Geometry: final body of the model. Coordinates: model frame, mm. Face numbers are marked on the shaded views. A direction names the side the tool comes from. Round coordinates to 2 decimals unless told otherwise and drop trailing zeros. Loops run counter-clockwise (first coordinate to the right, second up) from the corner with the lowest first, then second, coordinate; pieces in that order, holes last. Notation, with made-up numbers: (16.5, -19.5) - (36.5, -19.5) arc R23 cw to (36.5, 19.5) - close; hole circle Ø10 at (-13, 59). An arc over 180 degrees is marked (long way). Answer in a Markdown table with one row per item. Add a question column.
from build123d import *

# Parameters (mm, degrees)
CROQUIS2_W              = 82
CROQUIS2_H              = 82
CORTAR_EXTRUIR1_DEPTH   = 11.5
SALIENTE_EXTRUIR1_DEPTH = 10.5
CROQUIS4_W              = 14
CROQUIS4_H              = 8.5
CORTAR_EXTRUIR2_DEPTH   = 10.5
CROQUIS5_R              = 1.5
CORTAR_EXTRUIR3_DEPTH   = 10


with BuildPart() as part:
    # Croquis1 → Revolución1 (revolve)
    with BuildSketch(Plane.XY):
        Polygon((-67.901642817, 46.97611702), (-67.901642817, 61.97611702), (-67.901642817, 71.97611702), (-86.901642817, 71.97611702), (-86.901642817, 61.97611702), (-96.901642817, 61.97611702), (-96.901642817, 59.97611702), (-86.901642817, 59.97611702), (-69.901642817, 46.97611702), (-101.901642817, -33.02388298), (-99.901642817, -33.02388298), align=None)
    revolve(axis=Axis((-26.901642817, 46.97611702, 0), (0, -1, 0)))

    # Croquis2 → Cortar-Extruir1 (cut)
    with BuildSketch(Plane(origin=(0, 71.97611702, 0), x_dir=(1, 0, 0), z_dir=(0, 1, 0))):
        with Locations((-26.901642817, 0)):
            Rectangle(CROQUIS2_W, CROQUIS2_H)
    extrude(amount=-CORTAR_EXTRUIR1_DEPTH, mode=Mode.SUBTRACT)

    # Croquis3 → Saliente-Extruir1 (add)
    with BuildSketch(Plane(origin=(0, 71.97611702, 0), x_dir=(1, 0, 0), z_dir=(0, 1, 0))):
        with BuildLine():
            Line((32.419516983, 9), (25.098357183, 9))
            Line((25.098357183, 9), (25.098357183, -9))
            Line((25.098357183, -9), (32.419516983, -9))
            ThreePointArc((32.419516983, -9), (33.098357183, 0), (32.419516983, 9))
        make_face()
    extrude(amount=SALIENTE_EXTRUIR1_DEPTH)

    # Croquis4 → Cortar-Extruir2 (cut)
    with BuildSketch(Plane.ZY.offset(-25.098357183)):
        with Locations((0, 77.22611702)):
            Rectangle(CROQUIS4_W, CROQUIS4_H)
    extrude(amount=-CORTAR_EXTRUIR2_DEPTH, mode=Mode.SUBTRACT)

    # Croquis5 → Cortar-Extruir3 (cut)
    with BuildSketch(Plane(origin=(0, 61.97611702, 0), x_dir=(1, 0, 0), z_dir=(0, 1, 0))):
        with Locations((-26.901642817, -65)):
            Circle(CROQUIS5_R)
        with Locations((-83.193294063, 32.5)):
            Circle(CROQUIS5_R)
        with Locations((29.390008429, 32.5)):
            Circle(CROQUIS5_R)
    extrude(amount=-CORTAR_EXTRUIR3_DEPTH, mode=Mode.SUBTRACT)


solid = part.part
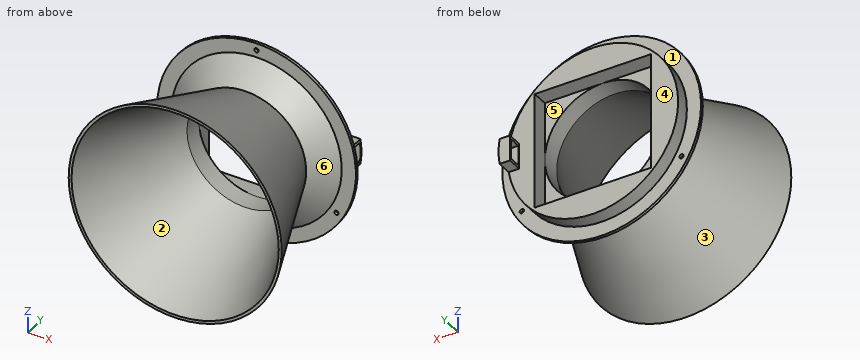
1) Pull-direction query (Z, two-part tool) for the marked faces 4, 5 and 6; classes: pulls with the +Z half, pulls with the -Z half, needs draft (parallel to the pull), parting line crosses it, or undercut.
2) Section A-A, the plane y = 51. Return the cut outline in (x, z), and give its area (3 significant figures).
3) Section B-B, the plane y = 2. Return the cut outline in (x, z), and give its area (3 significant figures).
4) Contact query for flat-ended pins moving along their axis: pin 1 Ø5 at (x, z) = (-83.19, -32.5) entering from +Y; pin 2 Ø2 at (y, z) = (58, 32.5) entering from +X; pin 3 Ø8 at (y, z) = (7, -31) entering from +X; pin 4 Ø6 at (x, y) = (-84.5, 51) entering from -Z. Output: stop coordinate, or through.
5) Material intervals for line 1 along X through (y, z) = (60.85, -32.5); line 2 along Y through (x, z) = (-62, 54.5); line 3 along Y through (x, z) = (25.5, -14), sorted ascending. Write a range as from..to.
6) Reachability of the marked faces 1, 2 and 3 from +Z, -Z, +X, -X, +Y, -Y: full face, straight path, thin tool, end or side. Return the list, or none.
Evaluation:
| question | item | result |
|---|---|---|
| 1 | face 4 | needs draft |
| 1 | face 5 | undercut |
| 1 | face 6 | parting line crosses it |
| 2 | outline | circle Ø96.52 at (-26.9, 0); hole circle Ø82 at (-26.9, 0) |
| 2 | area | 2,040 mm² |
| 3 | outline | circle Ø121.98 at (-26.9, 0); hole circle Ø117.98 at (-26.9, 0) |
| 3 | area | 754 mm² |
| 4 | pin 1 | stops at y = 61.98 |
| 4 | pin 2 | stops at x = 22.14 |
| 4 | pin 3 | stops at x = 26.22 |
| 4 | pin 4 | passes through |
| 5 | line 1 | x = -88.9..-84.69, -81.69..-67.9, 14.1..27.89, 30.89..35.1 |
| 5 | line 2 | y = -12.58..-7.58, 59.98..61.98 |
| 5 | line 3 | y = 13.88..18.88, 55.57..71.98 |
| 6 | face 1 | +Y |
| 6 | face 2 | -Y |
| 6 | face 3 | none |
